The figure shows three views and two pictorial views of one solid part (mm, origin at its lowest corner). Answer the questions. Coordinates: 2 decimals unless noted, no trailing zeros. Order: outer loops, then holes, each group sorted by start corner. A loop starts at its lowest first (then second) coordinate and runs counter-clockwise, first axis right, second up.
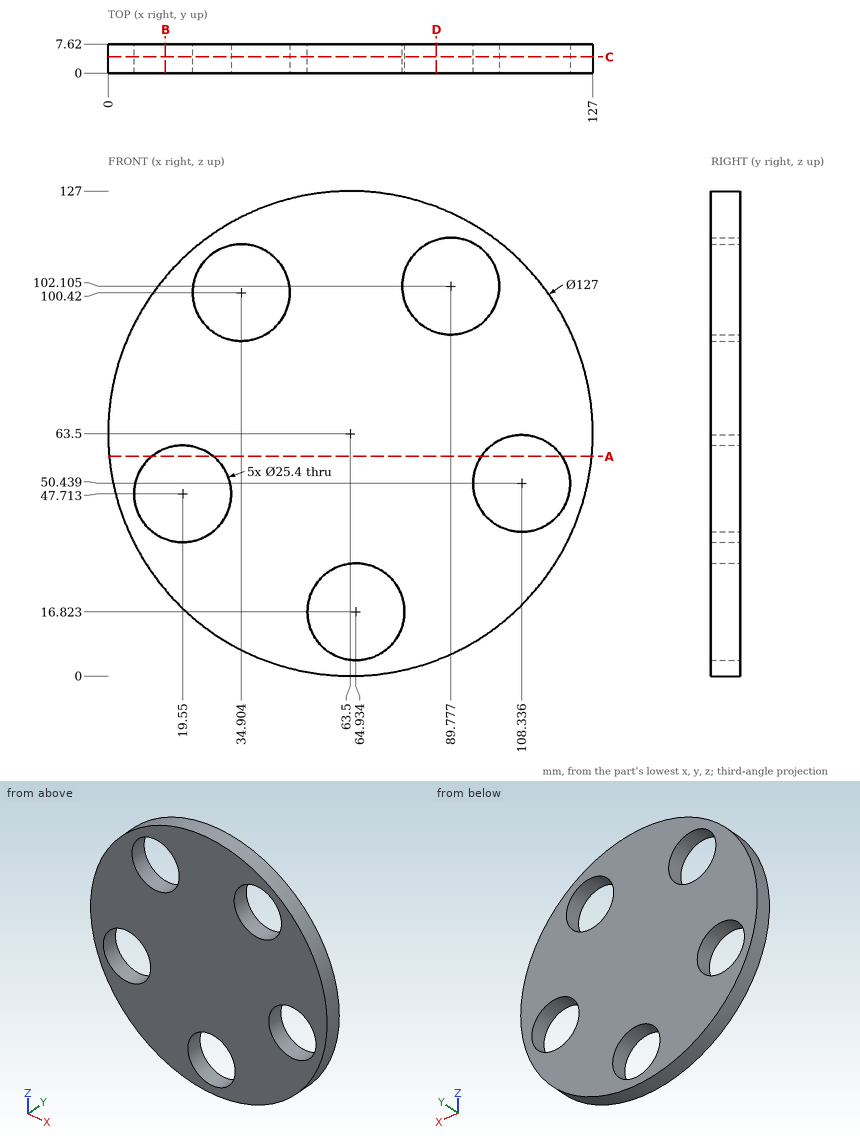
Q1. Straight lines are drawn through the part: L1, parallel to Z at x = 111, y = 0.5 (1 decimal); L2, parallel to Z at x = 41.5, y = 2.75 (1 decimal); L3, parallel to X at y = 1.25, z = 48. For each, find the intervals that lie inside material, in ascending order.
Q2. The part is cut by section D-D, the plane x = 86. Determine the outline of the cut face in (y, z), then the cut area to 3 significant figures.
Q3. Each of these flat-tipped pins is pushed along its axis until it touches: P1, Ø1, axis at y = 3, z = 93.5, coming from the -X side; P2, Ø4, axis at x = 50.5, z = 55.5, coming from the -Y side; P3, Ø1.5, axis at x = 69.5, y = 2, coming from the +Z side; P4, Ø1, axis at y = 4.5, z = 106.5, coming from the +X side. Where does it stop, or does it pass through?
Q4. The part is cut by section A-A, the plane z = 57.5. Determine the outline of the cut face in (x, y) (1 decimal), then the cut area to 3 significant figures.
Q5. The part is cut by section B-B, the plane x = 15. Determine the outline of the cut face in (y, z) (1 decimal), then the cut area to 3 significant figures.
Q6. The part is cut by section C-C, the plane y = 4.25. State how many separate pieces and enclosed holes the cut face has, then the cut area to 3 significant figures.
Computed values:
1. L1: z = 21.4 to 38, 62.9 to 105.6
1. L2: z = 3.9 to 89.6, 111.3 to 123.1
1. L3: x = 1.92 to 6.85, 32.25 to 95.87, 120.8 to 125.08
2. outline: (0, 4.12) - (7.62, 4.12) - (7.62, 89.98) - (0, 89.98) - close; (0, 114.23) - (7.62, 114.23) - (7.62, 122.88) - (0, 122.88) - close
2. area: 720 mm2
3. P1: stops at x = 7.27
3. P2: stops at y = 0
3. P3: stops at z = 126.78
3. P4: stops at x = 110.68
4. outline: (0.3, 0) - (11.5, 0) - (11.5, 7.6) - (0.3, 7.6) - close; (27.6, 0) - (97.8, 0) - (97.8, 7.6) - (27.6, 7.6) - close; (118.9, 0) - (126.7, 0) - (126.7, 7.6) - (118.9, 7.6) - close
4. area: 679 mm2
5. outline: (0, 22.5) - (7.6, 22.5) - (7.6, 35.9) - (0, 35.9) - close; (0, 59.6) - (7.6, 59.6) - (7.6, 104.5) - (0, 104.5) - close
5. area: 444 mm2
6. separate pieces: 1
6. enclosed holes: 5
6. area: 10,100 mm2
